```python
from build123d import *
from OCP.BRepFilletAPI import BRepFilletAPI_MakeChamfer

# Parameters (mm, degrees)
RESSALTO_EXTRUS_O1_DEPTH = 6
RESSALTO_EXTRUS_O2_DEPTH = 6
FILETE1_R                = 30
CHANFRO1_SIZE            = 2
CHANFRO1_SIZE2           = 5.464101615
FILETE2_R                = 2
RESSALTO_EXTRUS_O3_DEPTH = 6
FILETE3_R                = 2
CHANFRO2_SIZE            = 2


with BuildPart() as part:
    # Esboço1 → Ressalto-extrusão1 (new body)
    with BuildSketch(Plane.XY):
        Polygon((0, 0), (0, 65), (47, 65), (47, 53.693575035), (16, 0), align=None)
        Polygon((4.333825791, 50.65), (11.666174209, 50.65), (15.332348419, 57), (11.666174209, 63.35), (4.333825791, 63.35), (0.667651581, 57), align=None, mode=Mode.SUBTRACT)
        with BuildLine():
            Line((9, 20), (9, 10))
            ThreePointArc((9, 10), (6, 7), (3, 10))
            Line((3, 10), (3, 20))
            ThreePointArc((3, 20), (6, 23), (9, 20))
        make_face(mode=Mode.SUBTRACT)
        with BuildLine():
            Line((27, 62), (39, 62))
            ThreePointArc((39, 62), (42, 59), (39, 56))
            Line((39, 56), (27, 56))
            ThreePointArc((27, 56), (24, 59), (27, 62))
        make_face(mode=Mode.SUBTRACT)
    extrude(amount=RESSALTO_EXTRUS_O1_DEPTH)

    # Esboço2 → Ressalto-extrusão2 (add, through all)
    with BuildSketch(Plane.XY.offset(6)):
        Polygon((14.17764788, 65), (9.431163316, 73.221152423), (-11.093638754, 61.371152423), (0, 42.156406461), (0, 65), align=None)
    extrude(amount=-RESSALTO_EXTRUS_O2_DEPTH)

    # Filete1
    # the kernel refuses this fillet: 30 mm, written as the material it adds along each edge
    with BuildSketch(Plane(origin=(0, 42.156406461, 6), x_dir=(0, -1, 0), z_dir=(0, 0, -1))) as filete1_piece_1:
        with BuildLine():
            CenterArc((FILETE1_R * 0.267949192431, FILETE1_R), FILETE1_R, 240, 30)
            Line((-FILETE1_R * 0.232050807569, FILETE1_R * 0.133974596216), (-FILETE1_R * 0.242050807569, FILETE1_R * 0.11665408814))
            Line((-FILETE1_R * 0.242050807569, FILETE1_R * 0.11665408814), (-FILETE1_R * 0.00535898384862, -FILETE1_R * 0.02))
            Line((-FILETE1_R * 0.00535898384862, -FILETE1_R * 0.02), (FILETE1_R * 0.267949192431, -FILETE1_R * 0.02))
            Line((FILETE1_R * 0.267949192431, -FILETE1_R * 0.02), (FILETE1_R * 0.267949192431, 0))
        make_face()
    extrude(amount=6)
    with BuildSketch(Plane(origin=(14.17764788, 65, 6), x_dir=(1, 0, 0), z_dir=(0, 0, -1))) as filete1_piece_2:
        with BuildLine():
            CenterArc((15.885572973, -30), FILETE1_R, 90, 43.451100673)
            Line((-4.746484564, -8.221152423), (-5.159125715, -7.785575471))
            ThreePointArc((-5.159125715, -7.785575471), (-2.892857524, -3.810576211), (-0.519615242, 0.3))
            Line((-0.519615242, 0.3), (0, 0.6))
            Line((0, 0.6), (15.885572973, 0.6))
            Line((15.885572973, 0.6), (15.885572973, 0))
        make_face()
    extrude(amount=6)

    # Chanfro1: one chamfer whose edges measure the first distance from different faces: ONE call of the kernel's chamfer builder (chamfer() names one face for all edges)
    chanfro1_edges_1 = [part.edges().sort_by_distance(p)[0] for p in [
        (-11.093638754, 61.371152423, 3),
        (0, 0, 3),
        (47, 65, 3),
    ]]
    chanfro1_edges_2 = [part.edges().sort_by_distance(p)[0] for p in [
        (16, 0, 3),
    ]]
    chanfro1_side_2 = [part.faces().sort_by_distance(p)[0] for p in [
        (8, 0, 3),
    ]]
    chanfro1 = BRepFilletAPI_MakeChamfer(part.part.solid().wrapped)
    for e in chanfro1_edges_1:
        chanfro1.Add(CHANFRO1_SIZE, e.wrapped)
    for e in chanfro1_edges_2:
        chanfro1.Add(CHANFRO1_SIZE, CHANFRO1_SIZE2, e.wrapped, chanfro1_side_2[0].wrapped)  # the first distance lies on this face
    add(Compound.cast(chanfro1.Shape()), mode=Mode.REPLACE)

    # Filete2
    filete2_edges = [part.edges().sort_by_distance(p)[0] for p in [
        (9.431163316, 73.221152423, 3),
    ]]
    fillet(filete2_edges, radius=FILETE2_R)

    # Esboço3 → Ressalto-extrusão3 (add, through all)
    with BuildSketch(Plane.XY.offset(6)):
        Polygon((45, 65), (57, 65), (57, 53.693575035), (47, 53.693575035), (47, 63), align=None)
    extrude(amount=-RESSALTO_EXTRUS_O3_DEPTH)

    # Filete3
    filete3_edges = [part.edges().sort_by_distance(p)[0] for p in [
        (57, 65, 3),
        (47, 53.693575035, 3),
    ]]
    fillet(filete3_edges, radius=FILETE3_R)

    # Chanfro2
    chanfro2_edges = [part.edges().sort_by_distance(p)[0] for p in [
        (57, 53.693575035, 3),
    ]]
    chamfer(chanfro2_edges, length=CHANFRO2_SIZE)


solid = part.part
```
Part model, mm, in its own coordinate system. A direction names the side the tool comes from. Round coordinates to 2 decimals unless told otherwise and drop trailing zeros. Order: outer loops, then holes, each group sorted by start corner. A loop starts at its lowest first (then second) coordinate and runs counter-clockwise, first axis right, second up. Notation, with made-up numbers: M -14.5,80 L 30.5,80 A15 ccw 30.5,99 Z; hole C 45.5,21.5 d5. An arc over 180 degrees is marked long. Answer in a Markdown table with one row per item. Add a question column.
Q1. Pin check, flat tips, straight feed: pin 1 (1 mm diameter, centred on x = 39.5, z = 4.5, fed in from -Y); pin 2 (3 mm diameter, centred on x = 52, z = 2, fed in from -Y); pin 3 (3 mm diameter, centred on x = 35, z = 4, fed in from +Y). Stop position of each tip, or through.
Q2. 3-axis set-ups, long thin cutter, end or side, ignore diameter. For faces 4 (the face through (52, 53.694, 3)), 5 (the face through (-7.1, 54.45, 3.04)), 6 (the face through (13.525, 60.131, 2.958)): which of +Z, -Z, +X, -X, +Y, -Y reach the whole face in a straight line?
Q3. Cut at B-B on x = 37. Give the cut face in (y, z).
Q4. Cut at D-D on y = 19. Give the cut face in (x, z), and give its area (3 significant figures).
Q5. Cut at C-C on x = 6. Give the cut face in (y, z).
Q6. Wall check: L1, parallel to Y at x = 8.5, z = 3.1; L2, parallel to X at y = 59, z = 2.45; L3, parallel to X at y = 60, z = 4. Give the ranges that are in metal, low to high. Write a range as from..to.
Q7. Cut at A-A on z = 3.5. Give the number of separate pieces and of enclosed holes in the cut face, and give its area (3 significant figures).
Q8. Mould opens along Y. For faces 1 (the face through (57, 59, 3)), 2 (the face through (33, 62, 3)), 3 (the face through (19.756, 66.826, 3.042)) say: +Y half, -Y half, draft (parallel to the pull), parting line (faces both ways), or undercut.
Established:
| question | item | result |
|---|---|---|
| 1 | pin 1 | stops at y = 39.84 |
| 1 | pin 2 | stops at y = 53.69 |
| 1 | pin 3 | stops at y = 65 |
| 2 | face 4 | +Z, -Z, +X, -Y |
| 2 | face 5 | +Z, -Z, -X, -Y |
| 2 | face 6 | +Z, -Z |
| 3 | outline | M 36.37,0 L 56,0 L 56,6 L 36.37,6 Z; M 62,0 L 65,0 L 65,6 L 62,6 Z |
| 4 | outline | M 0,0 L 3,0 L 3,6 L 0,6 Z; M 9,0 L 26.97,0 L 26.97,6 L 9,6 Z |
| 4 | area | 126 mm2 |
| 5 | outline | M 0,0 L 7,0 L 7,6 L 0,6 Z; M 23,0 L 50.65,0 L 50.65,6 L 23,6 Z; M 63.35,0 L 71.24,0 L 71.24,6 L 63.35,6 Z |
| 6 | L1 | y = 0..8.34, 21.66..50.65, 63.35..72.65 |
| 6 | L2 | x = -9.72..1.82, 14.18..24, 42..57 |
| 6 | L3 | x = -10..2.4, 13.6..24.17, 41.83..57 |
| 7 | separate pieces | 1 |
| 7 | enclosed holes | 3 |
| 7 | area | 2,250 mm2 |
| 8 | face 1 | draft |
| 8 | face 2 | undercut |
| 8 | face 3 | +Y half |
